```python
from build123d import *

# Parameters (mm, degrees)
BOSS_EXTRUDE1_DEPTH = 3.175
SKETCH2_W           = 12.7
SKETCH2_H           = 3.175
BOSS_EXTRUDE2_DEPTH = 3.175
SKETCH3_W           = 3.175
SKETCH3_H           = 12.7
BOSS_EXTRUDE3_DEPTH = 3.175
CUT_EXTRUDE1_REACH  = 5.175
FILLET1_R           = 0.508


with BuildPart() as part:
    # Sketch1 → Boss-Extrude1 (new body)
    with BuildSketch(Plane.XY):
        with BuildLine():
            Line((22.86, -12.7), (-12.7, -12.7))
            add(Edge.make_bspline(
                [(22.86, 22.86), (14.060256121, 1.487897552), (8.672102448, -3.900256121), (-12.7, -12.7)],
                knots=[0, 0, 0, 0, 1, 1, 1, 1], degree=3))
            Line((22.86, 22.86), (22.86, -12.7))
        make_face()
    extrude(amount=BOSS_EXTRUDE1_DEPTH)

    # Sketch2 → Boss-Extrude2 (add)
    with BuildSketch(Plane.XZ.offset(12.7)):
        with Locations((3.81, 1.5875)):
            Rectangle(SKETCH2_W, SKETCH2_H)
    extrude(amount=BOSS_EXTRUDE2_DEPTH)

    # Sketch3 → Boss-Extrude3 (add)
    with BuildSketch(Plane(origin=(22.86, 0, 0), x_dir=(0, 0, -1), z_dir=(1, 0, 0))):
        with Locations((-1.5875, 6.35)):
            Rectangle(SKETCH3_W, SKETCH3_H)
    extrude(amount=BOSS_EXTRUDE3_DEPTH)

    # Sketch4 → Cut-Extrude1 (cut, up to next)
    with BuildSketch(Plane.XY.offset(3.175), mode=Mode.PRIVATE) as cut_extrude1_sk1:
        with BuildLine():
            Line((-3.556, -11.938), (-3.556, -12.7))
            Line((-3.556, -12.7), (-2.54, -12.7))
            Line((-2.54, -12.7), (-2.54, -11.938))
            ThreePointArc((-2.54, -11.938), (-3.048, -11.43), (-3.556, -11.938))
        make_face()
    cut_extrude1_tool1 = extrude(cut_extrude1_sk1.sketch, amount=-CUT_EXTRUDE1_REACH, mode=Mode.PRIVATE) & part.part
    add(cut_extrude1_tool1.solids().sort_by_distance((-3.048, -12.113972, 3.175))[0], mode=Mode.SUBTRACT)
    # Sketch4 → Cut-Extrude1 (cut, up to next)
    with BuildSketch(Plane.XY.offset(3.175), mode=Mode.PRIVATE) as cut_extrude1_sk2:
        with BuildLine():
            Line((10.16, -11.938), (10.16, -12.7))
            Line((10.16, -12.7), (11.176, -12.7))
            Line((11.176, -12.7), (11.176, -11.938))
            ThreePointArc((11.176, -11.938), (10.668, -11.43), (10.16, -11.938))
        make_face()
    cut_extrude1_tool2 = extrude(cut_extrude1_sk2.sketch, amount=-CUT_EXTRUDE1_REACH, mode=Mode.PRIVATE) & part.part
    add(cut_extrude1_tool2.solids().sort_by_distance((10.668, -12.113972, 3.175))[0], mode=Mode.SUBTRACT)
    # Sketch4 → Cut-Extrude1 (cut, up to next)
    with BuildSketch(Plane.XY.offset(3.175), mode=Mode.PRIVATE) as cut_extrude1_sk3:
        with BuildLine():
            Line((22.098, -1.016), (22.86, -1.016))
            Line((22.86, -1.016), (22.86, 0))
            Line((22.86, 0), (22.098, 0))
            ThreePointArc((22.098, 0), (21.59, -0.508), (22.098, -1.016))
        make_face()
    cut_extrude1_tool3 = extrude(cut_extrude1_sk3.sketch, amount=-CUT_EXTRUDE1_REACH, mode=Mode.PRIVATE) & part.part
    add(cut_extrude1_tool3.solids().sort_by_distance((22.273972, -0.508, 3.175))[0], mode=Mode.SUBTRACT)
    # Sketch4 → Cut-Extrude1 (cut, up to next)
    with BuildSketch(Plane.XY.offset(3.175), mode=Mode.PRIVATE) as cut_extrude1_sk4:
        with BuildLine():
            Line((22.098, 12.7), (22.86, 12.7))
            Line((22.86, 12.7), (22.86, 13.716))
            Line((22.86, 13.716), (22.098, 13.716))
            ThreePointArc((22.098, 13.716), (21.59, 13.208), (22.098, 12.7))
        make_face()
    cut_extrude1_tool4 = extrude(cut_extrude1_sk4.sketch, amount=-CUT_EXTRUDE1_REACH, mode=Mode.PRIVATE) & part.part
    add(cut_extrude1_tool4.solids().sort_by_distance((22.273972, 13.208, 3.175))[0], mode=Mode.SUBTRACT)

    # Fillet1
    fillet1_edges = [part.edges().sort_by_distance(p)[0] for p in [
        (22.86, 13.716, 1.5875),
        (26.035, 12.7, 1.5875),
        (26.035, 0, 1.5875),
        (22.86, -1.016, 1.5875),
        (22.86, -12.7, 1.5875),
        (11.176, -12.7, 1.5875),
        (10.16, -15.875, 1.5875),
        (-2.54, -15.875, 1.5875),
        (-3.556, -12.7, 1.5875),
        (-12.7, -12.7, 1.5875),
        (22.86, 22.86, 1.5875),
    ]]
    fillet(fillet1_edges, radius=FILLET1_R)


solid = part.part
```
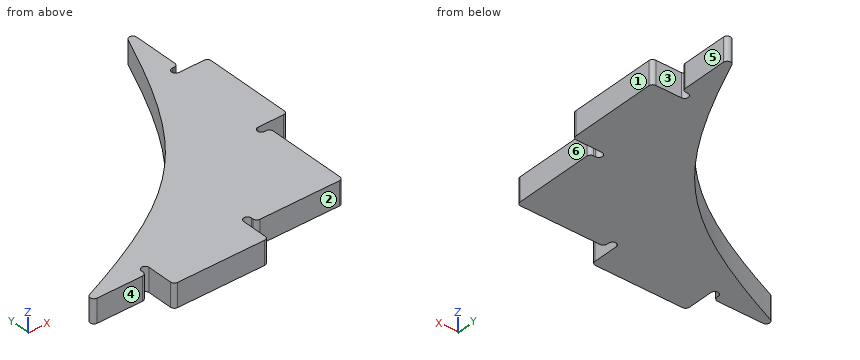
Model file for the job. Use its own axes, mm. Face numbers are marked on the shaded views. A direction names the side the tool comes from. Coordinates: 2 decimals unless noted, no trailing zeros. Answer as a JSON object with one key per item and string values. Group by question number.
1) Drill centre lines: L1, parallel to Y at x = 22.5, z = 1.8; L2, parallel to Y at x = 6.5, z = 1.85 (3 decimals); L3, parallel to Y at x = 10.5, z = 1.8. Where is each one in solid material? Low to high.
2) Which spindle directions (+Z, -Z, +X, -X, +Y, -Y) get a long thin tool onto all of the face, cutting with end or side? Do the marked faces 4, 5 and 6. Say none if no direction does.
3) Flat gauge pins, fed straight in: pin 1 (1 mm diameter, centred on x = 24, z = 2, fed in from +Y); pin 2 (1.5 mm diameter, centred on y = -2, z = 1.5, fed in from -X); pin 3 (1 mm diameter, centred on x = 18.5, z = 0.5, fed in from -Y). Where does each tip first touch, or does it go through?
4) Pull direction Y, two halves, no side cores. Call the marked faces 1, 2 and 3: +Y half, -Y half, draft (parallel to the pull), parting line (faces both ways), or undercut.
Check values:
{
 "1": {"L1": "y = -12.68 to -1.04, 0 to 12.7, 13.74 to 20.81", "L2": "y = -15.875 to -2.549", "L3": "y = -11.46 to 1.09"},
 "2": {"face 4": "+Z, -Z, -X, -Y", "face 5": "+Z, -Z, +X, +Y", "face 6": "+Z, -Z, +X, -Y"},
 "3": {"pin 1": "stops at y = 12.7", "pin 2": "stops at x = 6.24", "pin 3": "stops at y = -12.7"},
 "4": {"face 1": "draft", "face 2": "-Y half", "face 3": "undercut"}
}
